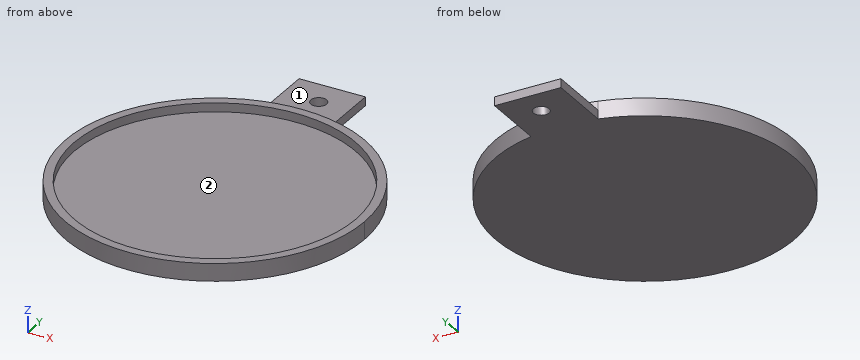
```python
from build123d import *

# Parameters (mm, degrees)
F0_R     = 40
F1_DEPTH = 5
F2_DEPTH = 2.5
F3_D     = 4.4958


with BuildPart() as f1:
    # F0 (on Top) → F1 (new body)
    with BuildSketch(Plane.XY):
        with BuildLine():
            ThreePointArc((-10.1377908892, 41.273177681), (-26.2239765025, -33.4447762198), (42.5, 0))
            ThreePointArc((42.5, 0), (32.9936503742, 26.7893455497), (8.7273395302, 41.5942729799))
            ThreePointArc((8.7273395302, 41.5942729799), (-0.7232695256, 42.4938452154), (-10.1377908892, 41.273177681))
        make_face()
        Circle(F0_R, mode=Mode.SUBTRACT)
    extrude(amount=F1_DEPTH)

    # F0 (on Top) → F2 (join)
    with BuildSketch(Plane.XY):
        with BuildLine():
            ThreePointArc((-10.1377908892, 41.273177681), (-0.7232695256, 42.4938452154), (8.7273395302, 41.5942729799))
            Line((8.7273395302, 41.5942729799), (8.7273395302, 59.7816915568))
            Line((8.7273395302, 59.7816915568), (-10.1377908892, 59.7816915568))
            Line((-10.1377908892, 59.7816915568), (-10.1377908892, 41.273177681))
        make_face()
        Circle(F0_R)
    extrude(amount=F2_DEPTH)

    # F3 (through all)
    with Locations(Plane(origin=(0, 0, 0), x_dir=(1, 0, 0), z_dir=(0, 0, -1))):
        with Locations((0, -51.7816915568)):
            Hole(F3_D / 2)


solid = f1.part
```
Geometry check sheet. Reference: the model listing, model coordinates, mm. Face numbers are marked on the shaded views. Coordinates: 2 decimals unless noted, no trailing zeros. Order: outer loops, then holes, each group sorted by start corner. A loop starts at its lowest first (then second) coordinate and runs counter-clockwise, first axis right, second up.
Item 1: Section check C-C (z = 3.9). Enter the section's corners in (x, y), plus the area to 3 significant figures.
Item 2: Section check B-B (y = 27.5). Enter the section's corners in (x, z).
Item 3: Mould release check, pull along X, two halves, no side actions. Record for the marked faces 1 and 2: released by +X, released by -X, zero draft, split by the parting line, or undercut.
Item 4: Scan lines: line 1 along Y through (x, z) = (0, 1.4); line 2 along Z through (x, y) = (21, -21); line 3 along X through (y, z) = (20, 4.4). Record each from-to range of solid material in increasing order.
Item 5: Section check D-D (x = -31.5). Enter the section's corners in (y, z).
Item 6: Section check A-A (x = 0). Enter the section's corners in (y, z).
Item 7: Depth check by flat-ended pin: pin 1 (2 mm diameter, centred on y = 52.5, z = 1, fed in from +X); pin 2 (2 mm diameter, centred on y = 15, z = 1.5, fed in from +X); pin 3 (3 mm diameter, centred on x = -15.5, y = -13, fed in from -Z); pin 4 (2 mm diameter, centred on y = 47, z = 1.5, fed in from -X). Enter the tip coordinate at first touch or a pass-through.
Check sheet entries:
1. outline: circle Ø85 at (0, 0); hole circle Ø80 at (0, 0)
1. area: 648 mm2
2. outline: (-32.4, 0) - (32.4, 0) - (32.4, 5) - (29.05, 5) - (29.05, 2.5) - (-29.05, 2.5) - (-29.05, 5) - (-32.4, 5) - close
3. face 1: zero draft
3. face 2: undercut
4. line 1: y = -42.5 to 49.53, 54.03 to 59.78
4. line 2: z = 0 to 2.5
4. line 3: x = -37.5 to -34.64, 34.64 to 37.5
5. outline: (-28.53, 0) - (28.53, 0) - (28.53, 5) - (24.65, 5) - (24.65, 2.5) - (-24.65, 2.5) - (-24.65, 5) - (-28.53, 5) - close
6. outline: (-42.5, 0) - (49.53, 0) - (49.53, 2.5) - (42.5, 2.5) - (42.5, 5) - (40, 5) - (40, 2.5) - (-40, 2.5) - (-40, 5) - (-42.5, 5) - close; (54.03, 0) - (59.78, 0) - (59.78, 2.5) - (54.03, 2.5) - close
7. pin 1: stops at x = 8.73
7. pin 2: stops at x = 40.13
7. pin 3: stops at z = 0
7. pin 4: stops at x = -10.14
